from build123d import *

# Parameters (mm, degrees)
F0_W            = 15
F0_H            = 26.25
F2_R            = 40
F2_R_2          = 26.25
F3_DEPTH        = 10
F4_R            = 3.5
F5_DEPTH        = 25.001
F5_COPIES_COUNT = 6


# Not quite as in the source:
# - a pattern or mirror of a feature is missing from the dataset's text; its kind, count and spacing are read off the source's solid


with BuildPart() as f1:
    # F0 (on Front) → F1 (revolve)
    with BuildSketch(Plane.XZ):
        with Locations((7.5, 13.125)):
            Rectangle(F0_W, F0_H)
    revolve(axis=Axis((-28.7704151153, 0, 0), (-1, 0, 0)))

    # F2 (on face) → F3 (join)
    with BuildSketch(Plane.YZ.offset(15)):
        Circle(F2_R)
        Circle(F2_R_2, mode=Mode.SUBTRACT)
        Circle(F2_R_2)
    extrude(amount=F3_DEPTH)

    # F4 (on face) → F5 (cut, through all)
    with BuildSketch(Plane(origin=(0, 0, 0), x_dir=(0, -1, 0), z_dir=(-1, 0, 0))):
        with Locations((30.3108891325, 17.5)):
            Circle(F4_R)
    f5 = extrude(amount=-F5_DEPTH, mode=Mode.SUBTRACT)

    # F5_copies: F5 ×6 about axis
    f5_copies_axis = Axis((0, 0, 0), (1, 0, 0))
    for i in range(1, F5_COPIES_COUNT):
        add(f5.rotate(f5_copies_axis, i * 360 / F5_COPIES_COUNT), mode=Mode.SUBTRACT)


solid = f1.part
Design review of the part built by this model. Coordinates are the model's own, in mm. A direction names the side the tool comes from. Give positions to 0.01 mm unless a question says otherwise; leave off trailing zeros. Loops run counter-clockwise (first coordinate to the right, second up) from the corner with the lowest first, then second, coordinate; pieces in that order, holes last. Notation, with made-up numbers: (3, 62) - (58, 62) arc R8 cw to (58, 66) - close; hole circle Ø9 at (-17.5, -6.75). An arc over 180 degrees is marked (long way). Use CSV: the item, a comma, the result in double quotes. Start each with the question number.
1. Insertion check: P1, Ø1, axis at x = 15, y = -4, coming from the -Z side; P2, Ø5, axis at x = 14.5, y = 10.5, coming from the +Z side; P3, Ø5, axis at y = -18, z = 23.5, coming from the -X side. Each pin has a flat end and moves straight along its axis. Give the tip position at first contact, or say it passes through.
2. Add section D-D (x = 22.5). State the section outline as (y, z) points.
3. Add section C-C (z = -35). State the section outline as (x, y) points, plus the area to 3 significant figures.
4. Draft analysis for pull direction Z (two halves, no side actions). For faces 1 (the cylindrical face through (19.93, -30.77, -20.97)), 2 (the flat face through (25, -1, 1)), 3 (the cylindrical face through (19.93, -8.67, -39.05)), state which applies: released by +Z, released by -Z, zero draft, split by the parting line, or undercut.
5. Wall thickness on L1, parallel to Z at x = 19, y = 0; L2, parallel to Z at x = 18.5, y = -2; L3, parallel to X at y = 29, z = 4: over which ranges is each line inside the solid? List them lowest first.
6. Add section A-A (y = 0). State the section outline as (x, z) points.
7. Machinability: for faces 4 (the cylindrical face through (19.93, 33.65, -18.55)), 5 (the cylindrical face through (8, 8, 25)), which of the approach directions +Z, -Z, +X, -X, +Y, -Y give a long, thin tool a straight path to every point of the face, cutting with its end or side? Answer none if there is none.
8. Add section B-B (z = -17.5). State the section outline as (x, y) points.
Results found:
1,P1,"stops at z = -39.85"
1,P2,"stops at z = 39.18"
1,P3,"stops at x = 15"
2,outline,"circle Ø80 at (0, 0); hole circle Ø7 at (-30.31, -17.5); hole circle Ø7 at (-30.31, 17.5); hole circle Ø7 at (0, -35); hole circle Ø7 at (0, 35); hole circle Ø7 at (30.31, -17.5); hole circle Ø7 at (30.31, 17.5)"
3,outline,"(15, -19.36) - (25, -19.36) - (25, -3.5) - (15, -3.5) - close; (15, 3.5) - (25, 3.5) - (25, 19.36) - (15, 19.36) - close"
3,area,"317 mm²"
4,face 1,"undercut"
4,face 2,"zero draft"
4,face 3,"split by the parting line"
5,L1,"z = -40 to -38.5, -31.5 to 31.5, 38.5 to 40"
5,L2,"z = -39.95 to -37.87, -32.13 to 32.13, 37.87 to 39.95"
5,L3,"x = 15 to 25"
6,outline,"(0, -26.25) - (15, -26.25) - (15, -31.5) - (25, -31.5) - (25, 31.5) - (15, 31.5) - (15, 26.25) - (0, 26.25) - close; (15, -40) - (25, -40) - (25, -38.5) - (15, -38.5) - close; (15, 38.5) - (25, 38.5) - (25, 40) - (15, 40) - close"
7,face 4,"+X, -X"
7,face 5,"-X"
8,outline,"(0, -19.57) - (15, -19.57) - (15, -26.81) - (25, -26.81) - (25, 26.81) - (15, 26.81) - (15, 19.57) - (0, 19.57) - close; (15, -35.97) - (25, -35.97) - (25, -33.81) - (15, -33.81) - close; (15, 33.81) - (25, 33.81) - (25, 35.97) - (15, 35.97) - close"
